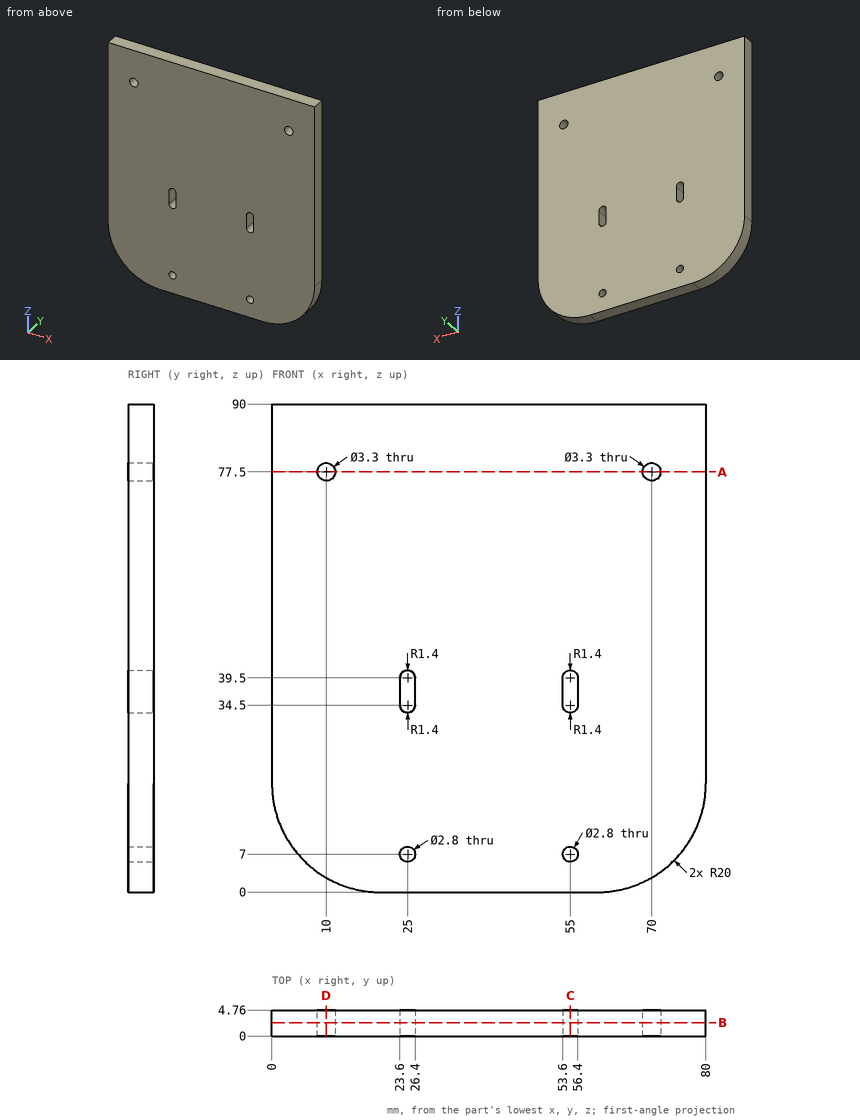
The drawing under review shows one solid part. Ordinate dimensions are in mm from its lowest x, y, z. Round coordinates to 2 decimals unless told otherwise and drop trailing zeros. Write each loop counter-clockwise with the first axis right and the second up, starting at its lowest first coordinate (ties: lowest second). Pieces come first, ordered by that corner, then holes. Notation, with made-up numbers: (76.25, -3.5) -> (118.25, -3.5) arc R15 ccw to (118.25, 16.5) -> close; hole circle Ø7 at (54.5, -17). An arc over 180 degrees is marked (long way). Put each result on its own line as item: value.
Q1. Consider section B-B on y = 2.45. State the section outline as (x, z) points, and give its area (3 significant figures).
Determined:
outline: (0, 20) arc R20 ccw to (20, 0) -> (60, 0) arc R20 ccw to (80, 20) -> (80, 90) -> (0, 90) -> close; hole circle Ø3.3 at (10, 77.5); hole circle Ø2.8 at (25, 7); hole (23.6, 34.5) arc R1.4 ccw to (26.4, 34.5) -> (26.4, 39.5) arc R1.4 ccw to (23.6, 39.5) -> close; hole circle Ø2.8 at (55, 7); hole (53.6, 34.5) arc R1.4 ccw to (56.4, 34.5) -> (56.4, 39.5) arc R1.4 ccw to (53.6, 39.5) -> close; hole circle Ø3.3 at (70, 77.5)
area: 6,960 mm^2
Q2. Clearance check with flat-ended pins moving along their axes: pin 1 Ø2 at (x, z) = (70, 77.5) entering from +Y; pin 2 Ø1 at (x, y) = (19, 2.5) entering from -Z. State where each tip first meets the part, or that it passes through.
Determined:
pin 1: passes through
pin 2: stops at z = 0.01
Q3. Consider section D-D on x = 10. State the section outline as (y, z) points, and give its area (3 significant figures).
Determined:
outline: (0, 2.68) -> (4.76, 2.68) -> (4.76, 75.85) -> (0, 75.85) -> close; (0, 79.15) -> (4.76, 79.15) -> (4.76, 90) -> (0, 90) -> close
area: 400 mm^2
Q4. Consider section A-A on z = 77.5. State the section outline as (x, y) points, and give its area (3 significant figures).
Determined:
outline: (0, 0) -> (8.35, 0) -> (8.35, 4.76) -> (0, 4.76) -> close; (11.65, 0) -> (68.35, 0) -> (68.35, 4.76) -> (11.65, 4.76) -> close; (71.65, 0) -> (80, 0) -> (80, 4.76) -> (71.65, 4.76) -> close
area: 349 mm^2
Q5. To check wall thickness, follow L1, parallel to X at y = 2.9, z = 77.5; L2, parallel to Z at x = 55, y = 3.25; L3, parallel to X at y = 3.7, z = 37. State the ranges of each line that lie inside material, in increasing order. Write a range as [from, to].
Determined:
L1: x = [0, 8.35], [11.65, 68.35], [71.65, 80]
L2: z = [0, 5.6], [8.4, 33.1], [40.9, 90]
L3: x = [0, 23.6], [26.4, 53.6], [56.4, 80]
Q6. Consider section C-C on x = 55. State the section outline as (y, z) points, and give its area (3 significant figures).
Determined:
outline: (0, 0) -> (4.76, 0) -> (4.76, 5.6) -> (0, 5.6) -> close; (0, 8.4) -> (4.76, 8.4) -> (4.76, 33.1) -> (0, 33.1) -> close; (0, 40.9) -> (4.76, 40.9) -> (4.76, 90) -> (0, 90) -> close
area: 378 mm^2
